from build123d import *

# Parameters (mm, degrees)
SKETCH1_R                      = 2.5
BOSS_EXTRUDE1_DEPTH            = 5
SKETCH7_R                      = 8
BOSS_EXTRUDE4_DEPTH            = 3
CBORE_FOR_M2_SHCS1_D           = 2.4
CBORE_FOR_M2_SHCS1_CBORE_D     = 4.4
CBORE_FOR_M2_SHCS1_CBORE_DEPTH = 2
SKETCH4_W                      = 34
SKETCH4_H                      = 23
BOSS_EXTRUDE2_DEPTH            = 7.5
SKETCH5_W                      = 7.5
SKETCH5_H                      = 4
SKETCH5_R                      = 1.2
BOSS_EXTRUDE3_DEPTH            = 2
CUT_EXTRUDE1_DEPTH             = 75.423192322
CUT_EXTRUDE1_DEPTH_BACK        = 75.423192322
SKETCH8_R                      = 3
SKETCH8_R_2                    = 1.2
BOSS_EXTRUDE5_DEPTH            = 2
FILLET4_R                      = 10
FILLET2_R                      = 20
FILLET3_R                      = 5
FILLET5_R                      = 7
CHAMFER4_SIZE                  = 2
CHAMFER1_SIZE                  = 1


with BuildPart() as part:
    # Sketch1 → Boss-Extrude1 (new body)
    with BuildSketch(Plane(origin=(0, 0, 0), x_dir=(0, 0, -1), z_dir=(1, 0, 0))):
        with BuildLine():
            ThreePointArc((0, 11.5), (-11.5, 0), (0, -11.5))
            Line((0, -11.5), (69.148836254, -11.5))
            Line((69.148836254, -11.5), (69.148836254, 11.5))
            Line((69.148836254, 11.5), (0, 11.5))
        make_face()
        Circle(SKETCH1_R, mode=Mode.SUBTRACT)
    extrude(amount=BOSS_EXTRUDE1_DEPTH)

    # Sketch7 → Boss-Extrude4 (add)
    with BuildSketch(Plane.ZY):
        Circle(SKETCH7_R)
    extrude(amount=BOSS_EXTRUDE4_DEPTH)

    # CBORE for M2 SHCS1 (through all)
    with Locations(Plane(origin=(5, 0, 0), x_dir=(0, 0, -1), z_dir=(1, 0, 0))):
        with Locations((-6, 0), (0, 6), (6, 0), (0, -6)):
            CounterBoreHole(CBORE_FOR_M2_SHCS1_D / 2, CBORE_FOR_M2_SHCS1_CBORE_D / 2, CBORE_FOR_M2_SHCS1_CBORE_DEPTH)

    # Sketch4 → Boss-Extrude2 (add)
    with BuildSketch(Plane.ZY):
        with Locations((-52.148836254, 0)):
            Rectangle(SKETCH4_W, SKETCH4_H)
    extrude(amount=BOSS_EXTRUDE2_DEPTH)

    # Sketch5 → Boss-Extrude3 (add)
    # profile 1 of 4: a face of its own
    with BuildSketch(Plane(origin=(0, 11.5, 0), x_dir=(1, 0, 0), z_dir=(0, 1, 0))):
        with Locations((-3.75, 37.148836254)):
            Rectangle(SKETCH5_W, SKETCH5_H)
    # profile 2 of 4: a face of its own
    with BuildSketch(Plane(origin=(0, 11.5, 0), x_dir=(1, 0, 0), z_dir=(0, 1, 0))):
        with BuildLine():
            Line((-7.5, 35.148836254), (-7.5, 39.148836254))
            Line((-7.5, 39.148836254), (-9.5, 39.148836254))
            ThreePointArc((-9.5, 39.148836254), (-11.5, 37.148836254), (-9.5, 35.148836254))
            Line((-9.5, 35.148836254), (-7.5, 35.148836254))
        make_face()
        with Locations(Location((-9.5, 37.148836254, 0), (0, 0, 270))):
            Circle(SKETCH5_R, mode=Mode.SUBTRACT)
    # profile 3 of 4: a face of its own
    with BuildSketch(Plane(origin=(0, 11.5, 0), x_dir=(1, 0, 0), z_dir=(0, 1, 0))):
        with Locations((-3.75, 67.148836254)):
            Rectangle(SKETCH5_W, SKETCH5_H)
    # profile 4 of 4: a face of its own
    with BuildSketch(Plane(origin=(0, 11.5, 0), x_dir=(1, 0, 0), z_dir=(0, 1, 0))):
        with BuildLine():
            Line((-7.5, 69.148836254), (-9.5, 69.148836254))
            ThreePointArc((-9.5, 69.148836254), (-11.5, 67.148836254), (-9.5, 65.148836254))
            Line((-9.5, 65.148836254), (-7.5, 65.148836254))
            Line((-7.5, 65.148836254), (-7.5, 69.148836254))
        make_face()
        with Locations(Location((-9.5, 67.148836254, 0), (0, 0, 270))):
            Circle(SKETCH5_R, mode=Mode.SUBTRACT)
    boss_extrude3 = extrude(amount=BOSS_EXTRUDE3_DEPTH)

    # Mirror1: Boss-Extrude3 across plane
    add(boss_extrude3.mirror(Plane.ZX))

    # Sketch6 → Cut-Extrude1 (cut, two sides: drawn at the far end of the back side and taken through both)
    with BuildSketch(Plane(origin=(0, 11.5, 0), x_dir=(1, 0, 0), z_dir=(0, 1, 0)).offset(-CUT_EXTRUDE1_DEPTH_BACK)):
        Polygon((-2.5, 69.148836254), (-2.5, 49.148836254), (5, 37.762357558), (5, 69.148836254), align=None)
    extrude(amount=CUT_EXTRUDE1_DEPTH + CUT_EXTRUDE1_DEPTH_BACK, mode=Mode.SUBTRACT)

    # Sketch8 → Boss-Extrude5 (add)
    # profile 1 of 2: a face of its own
    with BuildSketch(Plane(origin=(0, 13.5, 0), x_dir=(1, 0, 0), z_dir=(0, 1, 0))):
        with Locations((-9.5, 67.148836254)):
            Circle(SKETCH8_R)
        with Locations(Location((-9.5, 67.148836254, 0), (0, 0, 270))):
            Circle(SKETCH8_R_2, mode=Mode.SUBTRACT)
    # profile 2 of 2: a face of its own
    with BuildSketch(Plane(origin=(0, 13.5, 0), x_dir=(1, 0, 0), z_dir=(0, 1, 0))):
        with Locations((-9.5, 37.148836254)):
            Circle(SKETCH8_R)
        with Locations(Location((-9.5, 37.148836254, 0), (0, 0, 270))):
            Circle(SKETCH8_R_2, mode=Mode.SUBTRACT)
    boss_extrude5 = extrude(amount=-BOSS_EXTRUDE5_DEPTH)

    # Mirror2: Boss-Extrude5 across plane
    add(boss_extrude5.mirror(Plane.ZX))

    # Fillet4
    # the kernel refuses this fillet: 10 mm, written as the material it adds along each edge
    with BuildSketch(Plane(origin=(-7.263932023, 11.5, -69.148836254), x_dir=(-0.8150795156467411, 0, -0.5793491030225851), z_dir=(0, 1, 0))) as fillet4_piece_1:
        with BuildLine():
            CenterArc((3.540666656, -9.752076695), FILLET4_R, 102.784910078, 22.619864948)
            Line((-2.252824374, -1.601281538), (0, 0))
            ThreePointArc((0, 0), (0.663874998, -0.074376992), (1.327749996, 0))
        make_face()
    extrude(amount=2)
    with BuildSketch(Plane(origin=(-7.263932023, 11.5, -65.148836254), x_dir=(-0.8150795156467449, 0, 0.5793491030225799), z_dir=(0, 1, 0))) as fillet4_piece_2:
        with BuildLine():
            CenterArc((3.540666656, 9.752076695), FILLET4_R, 234.595224974, 22.619864948)
            Line((-2.252824374, 1.601281538), (0, 0))
            ThreePointArc((0, 0), (0.663874998, 0.074376992), (1.327749996, 0))
        make_face()
    extrude(amount=2)
    with BuildSketch(Plane(origin=(-7.263932023, 11.5, -35.148836254), x_dir=(1, 0, 0), z_dir=(0, 1, 0))) as fillet4_piece_3:
        with BuildLine():
            CenterArc((2.763932023, -10), FILLET4_R, 90, 22.619864948)
            ThreePointArc((-1.082221824, -0.769230769), (-0.498020668, -0.445238547), (0, 0))
            Line((0, 0), (2.763932023, 0))
        make_face()
    extrude(amount=2)
    with BuildSketch(Plane(origin=(-7.263932023, 11.5, -39.148836254), x_dir=(1, 0, 0), z_dir=(0, 1, 0))) as fillet4_piece_4:
        with BuildLine():
            CenterArc((2.763932023, 10), FILLET4_R, 247.380135052, 22.619864948)
            ThreePointArc((-1.082221824, 0.769230769), (-0.498020668, 0.445238547), (0, 0))
            Line((0, 0), (2.763932023, 0))
        make_face()
    extrude(amount=2)

    # Fillet2
    fillet2_edges = [part.edges().sort_by_distance(p)[0] for p in [
        (5, 0, -37.762357558),
        (-2.5, 0, -49.148836254),
    ]]
    fillet(fillet2_edges, radius=FILLET2_R)

    # Fillet3
    # the kernel refuses this fillet: 5 mm, written as the material it adds along each edge
    with BuildSketch(Plane(origin=(-4.5, 11.5, -65.148836254), x_dir=(0, 0, 1), z_dir=(1, 0, 0))) as fillet3_piece_1:
        with BuildLine():
            CenterArc((4, -5), FILLET3_R, 90, 53.130102354)
            Line((0, -2), (-0.08, -1.94))
            ThreePointArc((-0.08, -1.94), (-0.1, -1), (-0.1, 0))
            Line((-0.1, 0), (0, 0.1))
            Line((0, 0.1), (4, 0.1))
            Line((4, 0.1), (4, 0))
        make_face()
    extrude(amount=2)
    with BuildSketch(Plane(origin=(0, 11.5, -39.148836254), x_dir=(0, 0, -1), z_dir=(-1, 0, 0))) as fillet3_piece_2:
        with BuildLine():
            CenterArc((4, -5), FILLET3_R, 90, 53.130102354)
            Line((0, -2), (-0.08, -1.94))
            ThreePointArc((-0.08, -1.94), (-0.1, -1), (-0.1, 0))
            Line((-0.1, 0), (0, 0.1))
            Line((0, 0.1), (4, 0.1))
            Line((4, 0.1), (4, 0))
        make_face()
    extrude(amount=4.5)
    with BuildSketch(Plane(origin=(0, -11.5, -39.148836254), x_dir=(0, 0, -1), z_dir=(-1, 0, 0))) as fillet3_piece_3_section:
        with BuildLine():
            CenterArc((4, 5), FILLET3_R, 216.869897646, 53.130102354)
            Line((0, 2), (-0.08, 1.94))
            ThreePointArc((-0.08, 1.94), (-0.1, 1), (-0.1, 0))
            Line((-0.1, 0), (0, -0.1))
            Line((0, -0.1), (4, -0.1))
            Line((4, -0.1), (4, 0))
        make_face()
    fillet3_piece_3 = extrude(amount=17.263932023, mode=Mode.PRIVATE)
    fillet3_piece_3 = split(fillet3_piece_3, bisect_by=Plane(origin=(-7.5, -12.009955516, -40.183316128), z_dir=(1, 0, 0)), keep=Keep.TOP, mode=Mode.PRIVATE)
    add(fillet3_piece_3)
    with BuildSketch(Plane(origin=(-17.263932023, -11.5, -65.148836254), x_dir=(0, 0, 1), z_dir=(1, 0, 0))) as fillet3_piece_4_section:
        with BuildLine():
            CenterArc((4, 5), FILLET3_R, 216.869897646, 53.130102354)
            Line((0, 2), (-0.08, 1.94))
            ThreePointArc((-0.08, 1.94), (-0.1, 1), (-0.1, 0))
            Line((-0.1, 0), (0, -0.1))
            Line((0, -0.1), (4, -0.1))
            Line((4, -0.1), (4, 0))
        make_face()
    fillet3_piece_4 = extrude(amount=14.763932023, mode=Mode.PRIVATE)
    fillet3_piece_4 = split(fillet3_piece_4, bisect_by=Plane(origin=(-7.5, -12.00895453, -64.111805958), z_dir=(1, 0, 0)), keep=Keep.TOP, mode=Mode.PRIVATE)
    add(fillet3_piece_4)
    with BuildSketch(Plane(origin=(-4.5, 11.5, -55.148836254), x_dir=(0, 0, -1), z_dir=(1, 0, 0))) as fillet3_piece_5_section:
        with BuildLine():
            CenterArc((6, 5), FILLET3_R, 270, 53.130102354)
            Line((10, 2), (10.08, 1.94))
            ThreePointArc((10.08, 1.94), (10.1, 1), (10.1, 0))
            Line((10.1, 0), (10, -0.1))
            Line((10, -0.1), (6, -0.1))
            Line((6, -0.1), (6, 0))
        make_face()
    fillet3_piece_5 = revolve(axis=Axis((-4.5, 11.5, -55.148836254), (0, 1, 0)), revolution_arc=74.754248402, mode=Mode.PRIVATE)
    fillet3_piece_5 = split(fillet3_piece_5, bisect_by=Plane(origin=(-7.5, 12.098438569, -64.092030739), z_dir=(1, 0, 0)), keep=Keep.TOP, mode=Mode.PRIVATE)
    add(fillet3_piece_5)
    with BuildSketch(Plane(origin=(-4.5, 11.5, -49.148836254), x_dir=(-0.9648068245723973, 0, 0.2629596761074353), z_dir=(-0.2629596761074353, 0, -0.9648068245723973))) as fillet3_piece_6_section:
        with BuildLine():
            CenterArc((6, 5), FILLET3_R, 270, 53.130102354)
            Line((10, 2), (10.08, 1.94))
            ThreePointArc((10.08, 1.94), (10.1, 1), (10.1, 0))
            Line((10.1, 0), (10, -0.1))
            Line((10, -0.1), (6, -0.1))
            Line((6, -0.1), (6, 0))
        make_face()
    fillet3_piece_6 = revolve(axis=Axis((-4.5, 11.5, -49.148836254), (0, 1, 0)), revolution_arc=74.754248402, mode=Mode.PRIVATE)
    fillet3_piece_6 = split(fillet3_piece_6, bisect_by=Plane(origin=(-7.5, 12.098438572, -40.205641877), z_dir=(1, 0, 0)), keep=Keep.TOP, mode=Mode.PRIVATE)
    add(fillet3_piece_6)

    # Fillet5
    # the kernel refuses this fillet: 7 mm, written as the material it adds along each edge
    with BuildSketch(Plane(origin=(0, 11.5, -35.148836254), x_dir=(-1, 0, 0), z_dir=(0, -1, 0))) as fillet5_piece_1:
        with BuildLine():
            CenterArc((FILLET5_R, -FILLET5_R), FILLET5_R, 90, 90)
            Line((0, -FILLET5_R), (0, 0))
            Line((0, 0), (FILLET5_R, 0))
        make_face()
    extrude(amount=23)

    # Chamfer4
    chamfer4_edges = [part.edges().sort_by_distance(p)[0] for p in [
        (-2.5, 0, -69.148836254),
    ]]
    chamfer(chamfer4_edges, length=CHAMFER4_SIZE)

    # Chamfer1
    chamfer1_edges = [part.edges().sort_by_distance(p)[0] for p in [
        (5, 0, 11.5),
        (5, -11.5, -15.883704246),
        (5, 11.5, -15.883704246),
        (1.25, 11.5, -43.455596906),
        (1.25, -11.5, -43.455596906),
        (4.15785682, -11.5, -37.509927284),
        (4.15785682, 11.5, -37.509927284),
        (-1.65785682, 11.5, -49.401266528),
        (-1.65785682, -11.5, -49.401266528),
        (-2.5, 11.5, -58.146310787),
        (-2.5, -11.5, -58.146310787),
        (-2.5, -12.027864045, -63.384904232),
        (-2.5, 12.027864045, -63.384904232),
        (-2.5, 13.5, -66.148836254),
        (-2.5, -13.5, -66.148836254),
        (-3.5, 13.5, -68.148836254),
        (-3.5, -13.5, -68.148836254),
    ]]
    chamfer(chamfer1_edges, length=CHAMFER1_SIZE)


solid = part.part
Could you check a few things on this model? Use its own coordinates, in mm. A direction names the side the tool comes from. Give positions to 0.01 mm unless a question says otherwise; leave off trailing zeros. Loops run counter-clockwise (first coordinate to the right, second up) from the corner with the lowest first, then second, coordinate; pieces in that order, holes last. Notation, with made-up numbers: M 56.25,51 L 66.25,51 A20 ccw 66.25,79 Z; hole C -22.5,5.25 d7. An arc over 180 degrees is marked long. Answer as a JSON object with one key per item and string values.
Q1. Suppose I cut it at A-A, the plane x = -9.5. State how many separate pieces and enclosed holes the cut face has, plus the area to 3 significant figures.
Values found:
{"separate pieces": "8", "enclosed holes": "0", "area": "28.8 mm²"}
Q2. If we mould it in two halves opening along X, with no side actions, what happens to faces 6 (the cylindrical face through (4.014, 7.855, -1.183)), 7 (the cylindrical face through (-2.1, 0.16, -33.15)), 8 (the cylindrical face through (-9.447, 12.486, -38.348))? For each: pulls with the +X half, pulls with the -X half, needs draft (parallel to the pull), parting line crosses it, or undercut.
Values found:
{"face 6": "needs draft", "face 7": "pulls with the -X half", "face 8": "undercut"}
Q3. Suppose I cut it at D-D, the plane z = -26. List the corners of the cut face in (x, y) for me.
Values found:
{"outline": "M 0,-11.5 L 4,-11.5 L 5,-10.5 L 5,10.5 L 4,11.5 L 0,11.5 Z"}
Q4. If I drill on probe 1 along Y at (x, z) = (1.3, -6); probe 2 along X at (y, z) = (-4, -61); probe 3 along X at (y, z) = (3, -11.5), over which ranges is the centre line in solid material (lowest first)? Write a range as [from, to].
Values found:
{"probe 1": "y = [-11.5, -1.2], [1.2, 11.5]", "probe 2": "x = [-7.5, -2.5]", "probe 3": "x = [0, 5]"}
Q5. Suppose I cut it at C-C, the plane z = -6. List the corners of the cut face in (x, y) for me.
Values found:
{"outline": "M -3,-5.29 L 0,-5.29 L 0,-11.5 L 4,-11.5 L 5,-10.5 L 5,-2.2 L 3,-2.2 L 3,-1.2 L -3,-1.2 Z; M -3,1.2 L 3,1.2 L 3,2.2 L 5,2.2 L 5,10.5 L 4,11.5 L 0,11.5 L 0,5.29 L -3,5.29 Z"}
Q6. For P1, Ø3.5, axis at x = -6, y = -6.5, coming from the -Z side; P2, Ø1.6, axis at y = 12, z = -40, coming from the +X side; P3, Ø3, axis at y = 6, z = 0, coming from the +X side, each with a flat end and sliding along its axis, tell me the tip position at first contact or that it passes through.
Values found:
{"P1": "stops at z = -69.15", "P2": "stops at x = 2.53", "P3": "stops at x = 3"}
Q7. For faces 1 (the conical face through (-3.104, -11.658, -63.531)), 2 (the flat face through (0, -13, -38)), 3 (the flat face through (0, 12, -38)), 4 (the flat face through (3, 5, -1)), 5 (the flat face through (-2, 13, -35.149)), which set-ups out of +Z, -Z, +X, -X, +Y, -Y let a thin tool reach every point of the face, with its end or its side?
Values found:
{"face 1": "+X, -Y", "face 2": "+Z, -Z, +X, -Y", "face 3": "+Z, -Z, +X, +Y", "face 4": "+X", "face 5": "+Z, +X, +Y"}
